from build123d import *

# Parameters (mm, degrees)
F0_W     = 70
F0_H     = 70
F1_DEPTH = 1000
F2_W     = 70
F2_H     = 45
F3_DEPTH = 25
F4_W     = 45
F4_H     = 45
F5_DEPTH = 25
F6_W     = 70
F6_H     = 45
F7_DEPTH = 25
F8_W     = 45
F8_H     = 45
F9_DEPTH = 25


with BuildPart() as f1:
    # F0 (on Front) → F1 (new body)
    with BuildSketch(Plane.XZ):
        Rectangle(F0_W, F0_H)
    extrude(amount=-F1_DEPTH)

    # F2 (on face) → F3 (cut)
    with BuildSketch(Plane.XY.offset(35)):
        with Locations((0, 22.5)):
            Rectangle(F2_W, F2_H)
    extrude(amount=-F3_DEPTH, mode=Mode.SUBTRACT)

    # F4 (on face) → F5 (cut)
    with BuildSketch(Plane.YZ.offset(35)):
        with Locations((22.5, -12.5)):
            Rectangle(F4_W, F4_H)
    extrude(amount=-F5_DEPTH, mode=Mode.SUBTRACT)

    # F6 (on face) → F7 (cut)
    with BuildSketch(Plane.XY.offset(35)):
        with Locations((0, 897.5)):
            Rectangle(F6_W, F6_H)
    extrude(amount=-F7_DEPTH, mode=Mode.SUBTRACT)

    # F8 (on face) → F9 (cut)
    with BuildSketch(Plane.YZ.offset(35)):
        with Locations((897.5, -12.5)):
            Rectangle(F8_W, F8_H)
    extrude(amount=-F9_DEPTH, mode=Mode.SUBTRACT)


solid = f1.part
Model file for the job. Use its own axes, mm. A direction names the side the tool comes from. Round coordinates to 2 decimals unless told otherwise and drop trailing zeros. Loops run counter-clockwise (first coordinate to the right, second up) from the corner with the lowest first, then second, coordinate; pieces in that order, holes last. Notation, with made-up numbers: (3.5, -16.75) - (34.5, -16.75) arc R23 cw to (34.5, 12.25) - close; hole circle Ø7 at (58, 67). An arc over 180 degrees is marked (long way). Write each question's results on one line, items separated by ' | '.
(1) Saw through at C-C, the plane x = -21. List the corners of the cut face in (y, z), then the cut area to 4 significant figures.
Answer below:
outline: (0, -35) - (1000, -35) - (1000, 35) - (920, 35) - (920, 10) - (875, 10) - (875, 35) - (45, 35) - (45, 10) - (0, 10) - close | area: 67,750 mm^2
(2) Mould opens along Y. For faces 4 (the flat face through (10, 897, -12)), 5 (the flat face through (0, 1000, 0)), 6 (the flat face through (-35, 493, 0)) say: released by +Y, released by -Y, zero draft, split by the parting line, or undercut.
Answer below:
face 4: undercut | face 5: released by +Y | face 6: zero draft
(3) Saw through at A-A, the plane x = 20. List the corners of the cut face in (y, z), then the cut area to 3 significant figures.
Answer below:
outline: (45, -35) - (875, -35) - (875, 35) - (45, 35) - close; (920, -35) - (1000, -35) - (1000, 35) - (920, 35) - close | area: 63,700 mm^2
(4) Pin check, flat tips, straight feed: pin 1 (13.5 mm diameter, centred on y = 27, z = -16, fed in from +X); pin 2 (22.5 mm diameter, centred on x = -22, y = 898, fed in from +Z). Stop position of each tip, or through.
Answer below:
pin 1: stops at x = 10 | pin 2: stops at z = 10
(5) 3-axis set-ups, long thin cutter, end or side, ignore diameter. For faces 1 (the flat face through (7, 920, 16)), 2 (the flat face through (-13, 23, 10)), 3 (the flat face through (10, 22, -12)): which of +Z, -Z, +X, -X, +Y, -Y reach the whole face in a straight line?
Answer below:
face 1: +Z, +X | face 2: +Z, +X, -X, -Y | face 3: +Z, -Z, +X, -Y
(6) Saw through at B-B, the plane z = 1. List the corners of the cut face in (x, y), then the cut area to 4 significant figures.
Answer below:
outline: (-35, 0) - (10, 0) - (10, 45) - (35, 45) - (35, 875) - (10, 875) - (10, 920) - (35, 920) - (35, 1000) - (-35, 1000) - close | area: 67,750 mm^2
(7) Wall check: L1, parallel to Y at x = -6, z = 17; L2, parallel to X at y = 911, z = 0.5. Give the ranges that are in metal, low to high.
Answer below:
L1: y = 45 to 875, 920 to 1000 | L2: x = -35 to 10
